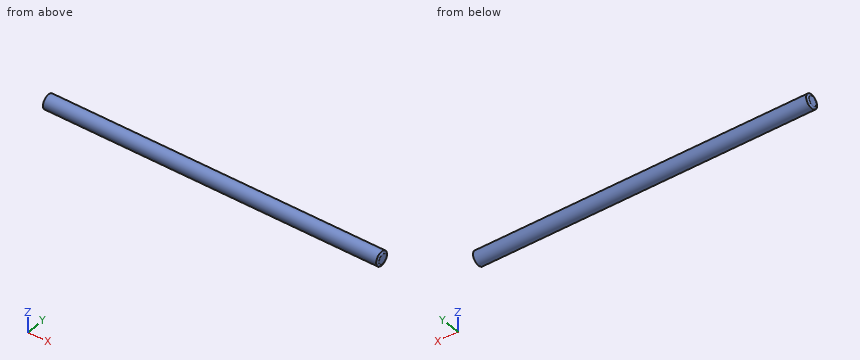
from build123d import *

# Parameters (mm, degrees)
F0_R       = 9
F1_DEPTH   = 425
F2_SIZE2   = 1.3989229745
F2_SIZE    = 3
F2_2_SIZE2 = 1.3989229745
F2_2_SIZE  = 3


with BuildPart() as f1:
    # F0 (on Right) → F1 (new body)
    with BuildSketch(Plane.YZ):
        Circle(F0_R)
    extrude(amount=F1_DEPTH)

    # F2
    f2_edges = [f1.edges().sort_by_distance(p)[0] for p in [
        (425, -9, 0),
    ]]
    f2_side = f1.faces().sort_by_distance((425, 0, 0))[0]
    chamfer(f2_edges, length=F2_SIZE, length2=F2_SIZE2, reference=f2_side)

    # F2#2
    f2_2_edges = [f1.edges().sort_by_distance(p)[0] for p in [
        (0, -9, 0),
    ]]
    f2_2_side = f1.faces().sort_by_distance((0, 0, 0))[0]
    chamfer(f2_2_edges, length=F2_2_SIZE, length2=F2_2_SIZE2, reference=f2_2_side)


solid = f1.part
Work out the finished part from the listing and answer in its coordinate system (mm). Coordinates: 2 decimals unless noted, no trailing zeros. Order: outer loops, then holes, each group sorted by start corner. A loop starts at its lowest first (then second) coordinate and runs counter-clockwise, first axis right, second up. Notation, with made-up numbers: (-19.5, 1) - (19.5, 1) arc R19 ccw to (19.5, 28) - close; hole circle Ø7 at (83.25, 74.25). An arc over 180 degrees is marked (long way). Put each result on its own line as item: value. Start each with the question number.
1) Find section A-A (x = 45.5). Give the vertices of the cut face in (y, z).
2) Find the intervals of material crossed by line 1 (X direction, y = -7.5, z = 4.75); line 2 (Y direction, x = 34.5, z = 6.75); line 3 (Y direction, x = 78.5, z = 0.75), in increasing order. Write a range as from..to.
3) Flat-ended cylindrical pins translate along their axes: pin 1 (1 mm diameter, centred on x = 163, y = 6, fed in from -Z); pin 2 (4 mm diameter, centred on x = 68.5, z = 5.5, fed in from -Y); pin 3 (2 mm diameter, centred on x = 89, y = 4, fed in from -Z). Find the tip coordinate at first contact, or state that the pin passes through.
Results list:
1. outline: circle Ø18 at (0, 0)
2. line 1: x = 1.34..423.66
2. line 2: y = -5.95..5.95
2. line 3: y = -8.97..8.97
3. pin 1: stops at z = -7.12
3. pin 2: stops at y = -8.29
3. pin 3: stops at z = -8.49
